Source: CAD feature listing. Evaluate the final solid. Frame: model axes, mm. Coordinates: 2 decimals unless noted, no trailing zeros. Order: outer loops, then holes, each group sorted by start corner. A loop starts at its lowest first (then second) coordinate and runs counter-clockwise, first axis right, second up.
Item 1: Ray query, line 1 (X direction, y = 31.5, z = 1.2); line 2 (Y direction, x = 75, z = 1.4); line 3 (X direction, y = 9.5, z = 1.8). Return the intervals inside material, ascending.
Item 2: Section B-B on y = 100. Return the cut outline in (x, z), then the cut area to 3 significant figures.
Item 3: Section A-A on z = 1.85. State how many separate pieces and enclosed holes the cut face has, then the cut area to 3 significant figures.
Item 4: Section C-C on y = 148. Return the cut outline in (x, z).
Item 5: Contact query for flat-ended pins moving along their axis: P1, Ø1.5, axis at y = 44.5, z = 1.5, coming from the -X side; P2, Ø0.9, axis at y = 29.5, z = 1.5, coming from the +X side; P3, Ø0.9, axis at x = 89.5, z = 1.5, coming from the -Y side. Output: stop coordinate, or through.
Item 6: Section D-D on x = -86. Return the cut outline in (y, z), then the cut area to 3 significant figures.
from build123d import *

# Parameters (mm, degrees)
SKETCH_2_R      = 10
SKETCH_2_R_2    = 1.5
EXTRUDE_2_DEPTH = 3


with BuildPart() as part:
    # 草图2 → 凸台-拉伸2 (new body)
    with BuildSketch(Plane.XY):
        with BuildLine():
            Line((-73, 0), (73, 0))
            ThreePointArc((73, 0), (77.949747468, 2.050252532), (80, 7))
            Line((80, 7), (80, 60))
            Line((80, 60), (105, 60))
            ThreePointArc((105, 60), (110.7284389, 62.976942983), (111.584524662, 69.375717782))
            Line((111.584524662, 69.375717782), (76.947414353, 165.375717782))
            ThreePointArc((76.947414353, 165.375717782), (74.385946708, 168.7284389), (70.362889691, 170))
            Line((70.362889691, 170), (-70.362889691, 170))
            ThreePointArc((-70.362889691, 170), (-74.385946708, 168.7284389), (-76.947414353, 165.375717782))
            Line((-76.947414353, 165.375717782), (-111.584524662, 69.375717782))
            ThreePointArc((-111.584524662, 69.375717782), (-110.7284389, 62.976942983), (-105, 60))
            Line((-105, 60), (-80, 60))
            Line((-80, 60), (-80, 7))
            ThreePointArc((-80, 7), (-77.949747468, 2.050252532), (-73, 0))
        make_face()
        with Locations((80, 100)):
            Circle(SKETCH_2_R, mode=Mode.SUBTRACT)
        with Locations((-72.441382232, 165.375717782)):
            Circle(SKETCH_2_R_2, mode=Mode.SUBTRACT)
        with Locations((-106.29148568, 65.75613767)):
            Circle(SKETCH_2_R_2, mode=Mode.SUBTRACT)
        with Locations(Location((106.29148568, 65.75613767, 0), (0, 0, 180))):
            Circle(SKETCH_2_R_2, mode=Mode.SUBTRACT)
        with Locations(Location((72.441382232, 165.375717782, 0), (0, 0, 180))):
            Circle(SKETCH_2_R_2, mode=Mode.SUBTRACT)
        with Locations((-75, 3.552033702)):
            Circle(SKETCH_2_R_2, mode=Mode.SUBTRACT)
        with Locations(Location((75, 3.552033702, 0), (0, 0, 180))):
            Circle(SKETCH_2_R_2, mode=Mode.SUBTRACT)
        with BuildLine():
            Line((-10, 22.5), (10, 22.5))
            ThreePointArc((10, 22.5), (13.535533906, 23.964466094), (15, 27.5))
            Line((15, 27.5), (15, 32.5))
            ThreePointArc((15, 32.5), (13.535533906, 36.035533906), (10, 37.5))
            Line((10, 37.5), (-10, 37.5))
            ThreePointArc((-10, 37.5), (-13.535533906, 36.035533906), (-15, 32.5))
            Line((-15, 32.5), (-15, 27.5))
            ThreePointArc((-15, 27.5), (-13.535533906, 23.964466094), (-10, 22.5))
        make_face(mode=Mode.SUBTRACT)
    extrude(amount=EXTRUDE_2_DEPTH)


solid = part.part
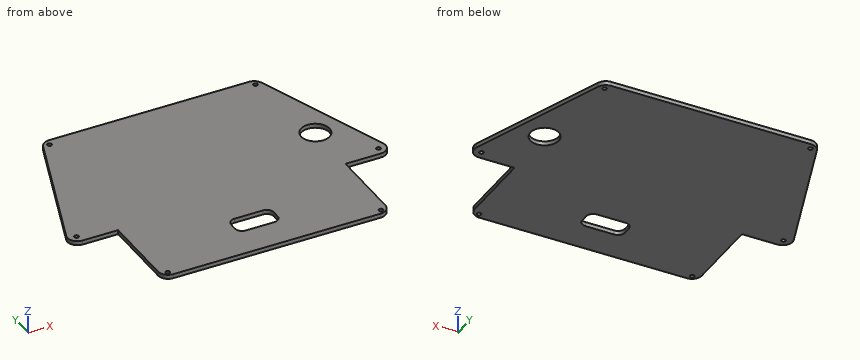
Answer list:
1. line 1: x = -80 to -15, 15 to 80
1. line 2: y = 0.29 to 2.05, 5.05 to 91.34, 108.66 to 168.24
1. line 3: x = -80 to 80
2. outline: (-100.54, 0) - (70, 0) - (70, 3) - (-100.54, 3) - close; (90, 0) - (100.54, 0) - (100.54, 3) - (90, 3) - close
2. area: 543 mm2
3. separate pieces: 1
3. enclosed holes: 8
3. area: 29,700 mm2
4. outline: (-83.22, 0) - (83.22, 0) - (83.22, 3) - (-83.22, 3) - close
5. P1: stops at x = -80
5. P2: stops at x = 80
5. P3: stops at y = 60
6. outline: (60, 0) - (140.29, 0) - (140.29, 3) - (60, 3) - close
6. area: 241 mm2
